Check sheet for the drawn part. Datum: minimum x, y, z corner. Units: mm. A direction names the side the tool comes from. Round coordinates to 2 decimals unless told otherwise and drop trailing zeros. Loops run counter-clockwise (first coordinate to the right, second up) from the corner with the lowest first, then second, coordinate; pieces in that order, holes last. Notation, with made-up numbers: (46, 54) - (87, 54) arc R22 cw to (87, 68) - close; hole circle Ø7 at (-13, -37). An arc over 180 degrees is marked (long way). Use CSV: the item, a comma, the result in double quotes.
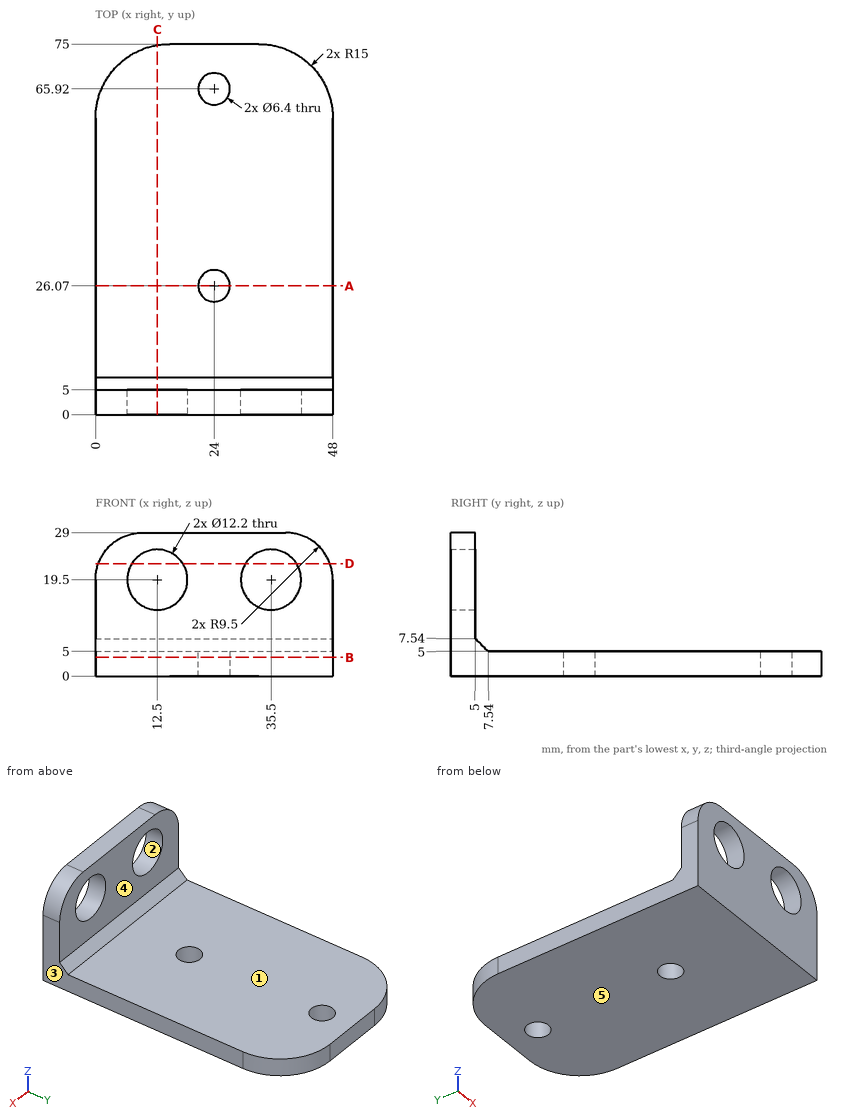
1) Cross-section at D-D, the plane z = 22.75. Record the cut outline in (x, y), then the cut area to 3 significant figures.
Returned:
outline,"(0.57, 0) - (7.34, 0) - (7.34, 5) - (0.57, 5) - close; (17.66, 0) - (30.34, 0) - (30.34, 5) - (17.66, 5) - close; (40.66, 0) - (47.43, 0) - (47.43, 5) - (40.66, 5) - close"
area,"131 mm²"
2) Access from +Z, -Z, +X, -X, +Y, -Y to the whole of each face (thin tool, end or side, straight path). Record for the marked faces 4 and 5.
Returned:
face 4,"+Z, +X, -X, +Y"
face 5,"-Z, +X, -X, +Y, -Y"
3) Gauge pin test, flat ends, axial feed: pin 1 Ø10 at (x, y) = (34.5, 54.5) entering from -Z; pin 2 Ø12 at (x, y) = (8.5, 40.5) entering from +Z. Record the tip position at first contact, or that the pin passes through.
Returned:
pin 1,"stops at z = 0"
pin 2,"stops at z = 5"
4) Thickness scan on probe 1 along Y at (x, z) = (24, 3.35); probe 2 along Z at (x, y) = (35.5, 3.55); probe 3 along Z at (x, y) = (33, 53). Record the ranges inside material, lowest first. Write a range as [from, to].
Returned:
probe 1,"y = [0, 22.87], [29.27, 62.72], [69.12, 75]"
probe 2,"z = [0, 13.4], [25.6, 29]"
probe 3,"z = [0, 5]"
5) Mould release check, pull along X, two halves, no side actions. Record for the marked faces 1, 2 and 3: +X half, -X half, draft (parallel to the pull), parting line (faces both ways), or undercut.
Returned:
face 1,"draft"
face 2,"undercut"
face 3,"+X half"
6) Cross-section at C-C, the plane x = 12.5. Record the cut outline in (y, z).
Returned:
outline,"(0, 0) - (74.79, 0) - (74.79, 5) - (7.54, 5) - (5, 7.54) - (5, 13.4) - (0, 13.4) - close; (0, 25.6) - (5, 25.6) - (5, 29) - (0, 29) - close"
7) Cross-section at B-B, the plane z = 3.75. Record the cut outline in (x, y), then the cut area to 3 significant figures.
Returned:
outline,"(0, 0) - (48, 0) - (48, 60) arc R15 ccw to (33, 75) - (15, 75) arc R15 ccw to (0, 60) - close; hole circle Ø6.4 at (24, 26.07); hole circle Ø6.4 at (24, 65.92)"
area,"3,440 mm²"
8) Cross-section at A-A, the plane y = 26.07. Record the cut outline in (x, z), then the cut area to 3 significant figures.
Returned:
outline,"(0, 0) - (20.8, 0) - (20.8, 5) - (0, 5) - close; (27.2, 0) - (48, 0) - (48, 5) - (27.2, 5) - close"
area,"208 mm²"
